```python
from build123d import *

# Parameters (mm, degrees)
F0_W     = 380
F0_H     = 360
F0_R     = 2.65
F0_W_2   = 336
F0_H_2   = 259
F1_DEPTH = 3


with BuildPart() as f1:
    # F0 (on Top) → F1 (new body)
    with BuildSketch(Plane.XY):
        Rectangle(F0_W, F0_H)
        with Locations((-180, -170)):
            Circle(F0_R, mode=Mode.SUBTRACT)
        with Locations((180, -170)):
            Circle(F0_R, mode=Mode.SUBTRACT)
        with Locations((0, -2.5)):
            Rectangle(F0_W_2, F0_H_2, mode=Mode.SUBTRACT)
        with Locations((-180, 170)):
            Circle(F0_R, mode=Mode.SUBTRACT)
        with Locations((180, 170)):
            Circle(F0_R, mode=Mode.SUBTRACT)
    extrude(amount=F1_DEPTH)


solid = f1.part
```
Read the model definition and answer for the solid it produces. Units are mm, in the model's axes. Coordinates: 2 decimals unless noted, no trailing zeros. Loops run counter-clockwise (first coordinate to the right, second up) from the corner with the lowest first, then second, coordinate; pieces in that order, holes last.
(1) The part is cut by section C-C (z = 2.05). Determine the outline of the cut face in (x, y), and give its area (3 significant figures).
Solution:
outline: (-190, -180) - (190, -180) - (190, 180) - (-190, 180) - close; hole circle Ø5.3 at (-180, -170); hole circle Ø5.3 at (-180, 170); hole (-168, -132) - (168, -132) - (168, 127) - (-168, 127) - close; hole circle Ø5.3 at (180, -170); hole circle Ø5.3 at (180, 170)
area: 49,700 mm2
(2) The part is cut by section B-B (y = 98.5). Determine the outline of the cut face in (x, z).
Solution:
outline: (-190, 0) - (-168, 0) - (-168, 3) - (-190, 3) - close; (168, 0) - (190, 0) - (190, 3) - (168, 3) - close
(3) The part is cut by section A-A (x = 85). Determine the outline of the cut face in (y, z), and give its area (3 significant figures).
Solution:
outline: (-180, 0) - (-132, 0) - (-132, 3) - (-180, 3) - close; (127, 0) - (180, 0) - (180, 3) - (127, 3) - close
area: 303 mm2
(4) A flat-ended cylindrical pin translates along its axis: pin 1 Ø5 at (x, y) = (180, 170) entering from +Z. Find the tip coordinate at first contact, or state that the pin passes through.
Solution:
pin 1: passes through
(5) Consider line 1 along X through (y, z) = (-170, 1.2); line 2 along Y through (x, z) = (-180, 2.35); line 3 along X through (y, z) = (9.5, 1.95). Determine where each line is inside the solid, lowest interval first.
Solution:
line 1: x = -190 to -182.65, -177.35 to 177.35, 182.65 to 190
line 2: y = -180 to -172.65, -167.35 to 167.35, 172.65 to 180
line 3: x = -190 to -168, 168 to 190
